Autodesk Inventor part; units mm, degrees
ref_plane "YZ Plane" through (0, 0, 0) normal (1, 0, 0) x (0, 1, 0)
ref_plane "XZ Plane" through (0, 0, 0) normal (0, 1, 0) x (-1, 0, 0)
ref_plane "XY Plane" through (0, 0, 0) normal (0, 0, 1) x (1, 0, 0)
sketch "Sketch1" plane through (0, 0, 0) normal (0, 1, 0) x (-1, 0, 0)
  line L0 (20, -10) -> (-20, -10)
  line L1 (-20, -10) -> (-20, 10)
  line L2 (-20, 10) -> (20, 10)
  line L3 (20, 10) -> (20, -10)
  line L4 (20, -10) -> (-20, 10) construction
  line L5 (-20, -10) -> (20, 10) construction
  point P0 (0, 0)
  dimension "d0" = 40
  dimension "d1" = 20
extrude "Extrusion1" add sketch "Sketch1" along normal blind 3.2
sketch "Sketch2" plane through (0, 0, 0) normal (0, -1, 0) x (1, 0, 0)
  line L0 (-20, -10) -> (20, -10)
  line L1 (-20, 10) -> (-20, -10)
  point P0 (0, 0)
  point P1 (-10, 0)
  point P2 (10, 0)
  dimension "d4" = 10
  dimension "d5" = 20
  dimension "d6" = 10
hole "Hole1" at (-10, 0, 0) at (10, 0, 0) direction (0, 1, 0) diameter 5 end through all counterbore diameter 9 counterbore depth 1.5
sketch "Sketch3" plane through (0, 3.2, 0) normal (0, 1, 0) x (1, 0, 0)
  line L0 (-20, -10) -> (20, -10)
  line L1 (2.3776, -5.74) -> (-2.3776, -5.74)
  line L2 (-2.3776, -5.74) -> (-5.74, -2.3776)
  line L3 (-5.74, -2.3776) -> (-5.74, 2.3776)
  line L4 (-5.74, 2.3776) -> (-2.3776, 5.74)
  line L5 (-2.3776, 5.74) -> (2.3776, 5.74)
  line L6 (2.3776, 5.74) -> (5.74, 2.3776)
  line L7 (5.74, 2.3776) -> (5.74, -2.3776)
  line L8 (5.74, -2.3776) -> (2.3776, -5.74)
  point P0 (0, 0)
  point P1 (0, 0)
  dimension "d14" = 11.48
extrude "Extrusion2" add sketch "Sketch3" along normal blind 9.5
sketch "Sketch4" plane through (0, 12.7, 0) normal (0, 1, 0) x (1, 0, 0)
  point P0 (0, 0)
  point P1 (0, 0)
hole "Hole2" at (0, 12.7, 0) direction (0, -1, 0) diameter 6.647 end through all
fillet "Fillet1" radius 1.5 4 edges at (-20, 1.6, 10) (20, 1.6, 10) (20, 1.6, -10) (-20, 1.6, -10)
properties part number "Metric 8mm ACME Nut Plate" material "Acetal Resin, Black"
Can you work these out from the model? Positions are in its coordinate system, mm. A direction names the side the tool comes from. Give positions to 0.01 mm unless a question says otherwise; leave off trailing zeros. Loops run counter-clockwise (first coordinate to the right, second up) from the corner with the lowest first, then second, coordinate; pieces in that order, holes last. Notation, with made-up numbers: M 53.25,71 L 104.25,71 A24 cw 104.25,88 Z; hole C 80.25,7.5 d6. An arc over 180 degrees is marked long. One line per question, with ' | ' between items. Start each with the question number.
Q1. If I drill on line 1 (X direction, y = 2.7, z = 0); line 2 (Z direction, x = -10, y = 2.6); line 3 (Z direction, x = -10, y = 0.5), over which ranges is the centre line in solid material (lowest first)? Write a range as from..to.
Q2. If we section it at B-B (z = 0): Please give me the cut outline in (x, y), plus the area to 3 significant figures.
Q3. If we section it at A-A (x = -10): Please give me the cut outline in (y, z).
Q4. If we section it at C-C (y = 2.25): Please give me the cut outline in (x, z), plus the area to 3 significant figures.
Q5. If we section it at D-D (y = 11.25): Please give me the cut outline in (x, z), plus the area to 3 significant figures.
Q6. For faces 1 (the flat face through (-4.04, 7.88, 4.08)), 2 (the cylindrical face through (14.39, 0.76, 0.98)), 3 (the flat face through (0, 8, -5.74)), 4 (the flat face through (-4.08, 7.88, -4.04)), which set-ups out of +Z, -Z, +X, -X, +Y, -Y let a thin tool reach every point of the face, with its end or its side?
Q7. If we mould it in two halves opening along Z, with no side actions, what happens to faces 5 (the flat face through (-8, 1.5, -2)), 6 (the cylindrical face through (1.27, 6.26, 3.07)), 7 (the flat face through (0, 2, -10)), 8 (the flat face through (4.08, 7.88, 4.04))? For each: +Z half, -Z half, draft (parallel to the pull), parting line (faces both ways), or undercut.
Q8. For pin 1 Ø6 at (x, z) = (-10, 0) entering from +Y; pin 2 Ø1.4 at (y, z) = (8.5, -1) entering from -X; pin 3 Ø5 at (x, y) = (-0.5, 9) entering from -Z, each with a flat end and sliding along its axis, tell me the tip position at first contact or that it passes through.
Computed:
1) line 1: x = -20..-12.5, -7.5..-3.32, 3.32..7.5, 12.5..20 | line 2: z = -10..-2.5, 2.5..10 | line 3: z = -10..-4.5, 4.5..10
2) outline: M -20,0 L -14.5,0 L -14.5,1.5 L -12.5,1.5 L -12.5,3.2 L -20,3.2 Z; M -7.5,1.5 L -5.5,1.5 L -5.5,0 L -3.32,0 L -3.32,12.7 L -5.74,12.7 L -5.74,3.2 L -7.5,3.2 Z; M 3.32,0 L 5.5,0 L 5.5,1.5 L 7.5,1.5 L 7.5,3.2 L 5.74,3.2 L 5.74,12.7 L 3.32,12.7 Z; M 12.5,1.5 L 14.5,1.5 L 14.5,0 L 20,0 L 20,3.2 L 12.5,3.2 Z | area: 109 mm²
3) outline: M 0,-10 L 3.2,-10 L 3.2,-2.5 L 1.5,-2.5 L 1.5,-4.5 L 0,-4.5 Z; M 0,4.5 L 1.5,4.5 L 1.5,2.5 L 3.2,2.5 L 3.2,10 L 0,10 Z
4) outline: M -20,-8.5 A1.5 ccw -18.5,-10 L 18.5,-10 A1.5 ccw 20,-8.5 L 20,8.5 A1.5 ccw 18.5,10 L -18.5,10 A1.5 ccw -20,8.5 Z; hole C -10,0 d5; hole C 0,0 d6.65; hole C 10,0 d5 | area: 724 mm²
5) outline: M -5.74,-2.38 L -2.38,-5.74 L 2.38,-5.74 L 5.74,-2.38 L 5.74,2.38 L 2.38,5.74 L -2.38,5.74 L -5.74,2.38 Z; hole C 0,0 d6.65 | area: 74.5 mm²
6) face 1: +Z, -X, +Y | face 2: -Y | face 3: -Z, +X, -X, +Y | face 4: -Z, -X, +Y
7) face 5: undercut | face 6: undercut | face 7: -Z half | face 8: +Z half
8) pin 1: stops at y = 3.2 | pin 2: stops at x = -5.74 | pin 3: stops at z = -5.74
